Geometry check sheet. Reference: the model listing, model coordinates, mm. Give positions to 0.01 mm unless a question says otherwise; leave off trailing zeros. Loops run counter-clockwise (first coordinate to the right, second up) from the corner with the lowest first, then second, coordinate; pieces in that order, holes last. Notation, with made-up numbers: (-28.75, 72) -> (-18.75, 72) arc R36 ccw to (-18.75, 106) -> close; hole circle Ø10 at (70.25, -33). An arc over 180 degrees is marked (long way). Write item = value, one per line.
```python
from build123d import *

# Parameters (mm, degrees)
F0_R          = 13.25
F1_DEPTH      = 210
F3_DEPTH      = 11.5
F4_R          = 6.25
F5_DEPTH      = 210.001
F9_DEPTH      = 13.251
F9_DEPTH_BACK = 13.251


with BuildPart() as f1:
    # F0 (on Front) → F1 (new body)
    with BuildSketch(Plane.XZ):
        Circle(F0_R)
    extrude(amount=F1_DEPTH)

    # F2 (on face) → F3 (cut)
    with BuildSketch(Plane.XZ.offset(210)):
        with BuildLine():
            ThreePointArc((8.3964278119, 10.25), (0, 13.25), (-8.3964278119, 10.25))
            Line((-8.3964278119, 10.25), (8.3964278119, 10.25))
        make_face()
    extrude(amount=-F3_DEPTH, mode=Mode.SUBTRACT)

    # F4 (on face) → F5 (cut, through all)
    with BuildSketch(Plane.XZ.offset(210)):
        Circle(F4_R)
    extrude(amount=-F5_DEPTH, mode=Mode.SUBTRACT)

    # F6 (on Right) → F7 (revolve, cut)
    with BuildSketch(Plane.YZ):
        Polygon((-210, -15.6165892258), (-206, -13.25), (-210, -11.25), align=None)
    revolve(axis=Axis((0, -105, 0), (0, -1, 0)), mode=Mode.SUBTRACT)

    # F8 (on Right) → F9 (cut, two sides)
    with BuildSketch(Plane.YZ) as f9_sk:
        Polygon((-209.0051316588, 13.25), (-210, 13.25), (-210, -13.25), align=None)
    extrude(amount=-F9_DEPTH, mode=Mode.SUBTRACT)
    extrude(f9_sk.sketch, amount=F9_DEPTH_BACK, mode=Mode.SUBTRACT)

    # F10: F1 across plane


with BuildPart() as f1_1:
    add(f1.part)
    add(f1.part.mirror(Plane.XZ))


solid = f1_1.part
```
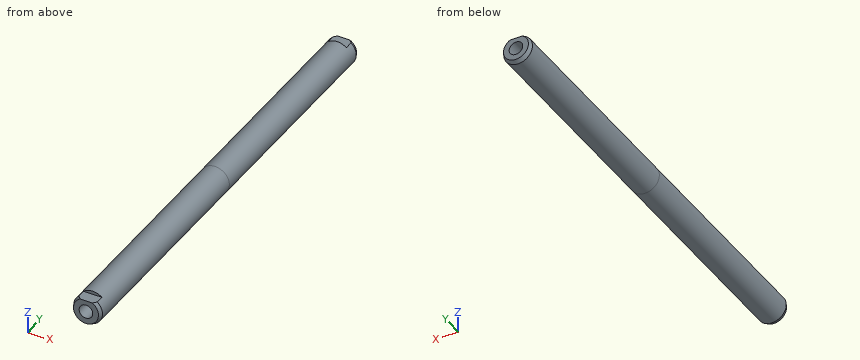
Item 1: Thickness scan on L1, parallel to Z at x = 0, y = -127.5; L2, parallel to Z at x = 3, y = 189.5. Record the ranges inside material, lowest first. Write a range as [from, to].
Answer:
L1 = [-13.25, -6.25], [6.25, 13.25]
L2 = [-12.91, -5.48], [5.48, 12.91]
Item 2: Section check B-B, the plane y = 46. Record the cut outline in (x, z), plus the area to 3 significant figures.
Answer:
outline = circle Ø26.5 at (0, 0); hole circle Ø12.5 at (0, 0)
area = 429 mm^2
Item 3: Section check A-A, the plane x = 0. Record the cut outline in (y, z).
Answer:
outline = (-209.93, -11.29) -> (-206, -13.25) -> (206, -13.25) -> (209.93, -11.29) -> (209.74, -6.25) -> (-209.74, -6.25) -> close; (-209.27, 6.25) -> (209.27, 6.25) -> (209.12, 10.25) -> (198.5, 10.25) -> (198.5, 13.25) -> (-198.5, 13.25) -> (-198.5, 10.25) -> (-209.12, 10.25) -> close
Item 4: Section check C-C, the plane z = 0. Record the cut outline in (x, y).
Answer:
outline = (-13.25, -206) -> (-11.5, -209.5) -> (-6.25, -209.5) -> (-6.25, 209.5) -> (-11.5, 209.5) -> (-13.25, 206) -> close; (6.25, -209.5) -> (11.5, -209.5) -> (13.25, -206) -> (13.25, 206) -> (11.5, 209.5) -> (6.25, 209.5) -> close
Item 5: Gauge pin test, flat ends, axial feed: pin 1 (10 mm diameter, centred on y = -101.5, z = -8, fed in from -X); pin 2 (10 mm diameter, centred on y = -139, z = -2, fed in from -X); pin 3 (0.9 mm diameter, centred on x = 2.5, z = 12, fed in from -Y); pin 4 (11.5 mm diameter, centred on x = -1.5, y = -206, fed in from +Z). Record the tip position at first contact, or that the pin passes through.
Answer:
pin_1 = -12.91
pin_2 = -13.25
pin_3 = -198.5
pin_4 = 10.25
